Source: three-view drawing plus pictorial views. Frame: mm from the lowest corner of the part. Coordinates: 2 decimals unless noted, no trailing zeros. Loops run counter-clockwise (first coordinate to the right, second up) from the corner with the lowest first, then second, coordinate; pieces in that order, holes last. Notation, with made-up numbers: M -12.5,-10.75 L 31.5,-10.75 A11 ccw 31.5,0.25 Z; hole C -18,62.5 d7. An arc over 180 degrees is marked long. Use a Markdown table: item, result. Add a question column.
1. Line query: L1, parallel to Y at x = 10, z = 19.55; L2, parallel to X at y = 190, z = 19.35; L3, parallel to X at y = 178, z = 9.25. Output: solid intervals per line, ascending. Write a range as [from, to].
2. Pin query (flat end, axial travel): pin 1 (5 mm diameter, centred on y = 80.5, z = 13.5, fed in from -X); pin 2 (5 mm diameter, centred on x = 5, y = 129, fed in from -Z); pin 3 (0.8 mm diameter, centred on x = 0.5, z = 12.5, fed in from -Y); pin 4 (3 mm diameter, centred on x = 10, y = 190, fed in from -Z). Return the tip coordinate at first contact, or that it passes through.
3. Section A-A on x = 10. Output: boundary loops of the cut face in (y, z), then the cut area to 4 significant figures.
4. Section B-B on y = 10. Output: boundary loops of the cut face in (x, z).
5. Section D-D on z = 7.75. Output: boundary loops of the cut face in (x, y).
6. Section C-C on y = 32. Output: boundary loops of the cut face in (x, z), then the cut area to 4 significant figures.
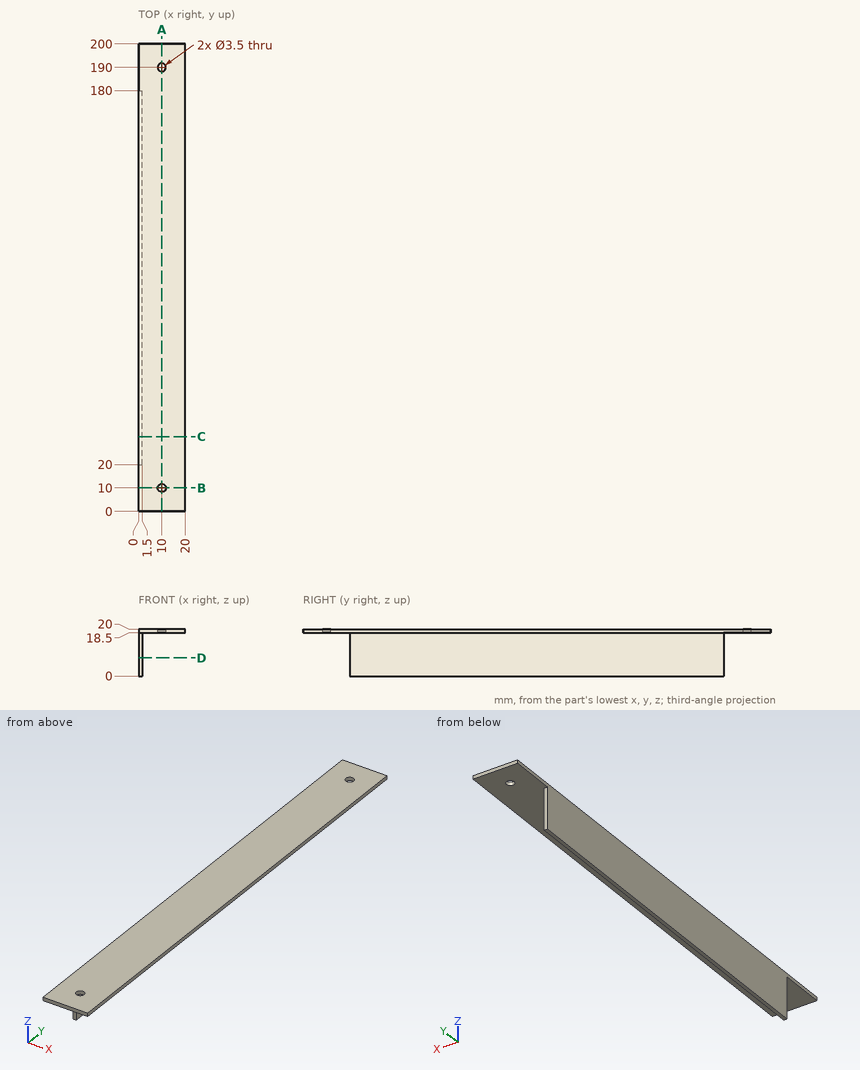
Answers below:
| question | item | result |
|---|---|---|
| 1 | L1 | y = [0, 8.25], [11.75, 188.25], [191.75, 200] |
| 1 | L2 | x = [0, 8.25], [11.75, 20] |
| 1 | L3 | x = [0, 1.5] |
| 2 | pin 1 | stops at x = 0 |
| 2 | pin 2 | stops at z = 18.5 |
| 2 | pin 3 | stops at y = 20 |
| 2 | pin 4 | passes through |
| 3 | outline | M 0,18.5 L 8.25,18.5 L 8.25,20 L 0,20 Z; M 11.75,18.5 L 188.25,18.5 L 188.25,20 L 11.75,20 Z; M 191.75,18.5 L 200,18.5 L 200,20 L 191.75,20 Z |
| 3 | area | 289.5 mm² |
| 4 | outline | M 0,18.5 L 8.25,18.5 L 8.25,20 L 0,20 Z; M 11.75,18.5 L 20,18.5 L 20,20 L 11.75,20 Z |
| 5 | outline | M 0,20 L 1.5,20 L 1.5,180 L 0,180 Z |
| 6 | outline | M 0,0 L 1.5,0 L 1.5,18.5 L 20,18.5 L 20,20 L 0,20 Z |
| 6 | area | 57.75 mm² |
